```python
from build123d import *

# Parameters (mm, degrees)
F0_W     = 40
F0_H     = 30
F1_DEPTH = 7.5
F2_W     = 21.86022
F2_H     = 7.61192
F3_DEPTH = 25
F4_R     = 1.8
F5_DEPTH = 20


with BuildPart() as f1:
    # F0 (on Top) → F1 (new body, symmetric)
    with BuildSketch(Plane.XY):
        Rectangle(F0_W, F0_H)
    extrude(amount=F1_DEPTH, both=True)

    # F2 (on face) → F3 (cut)
    with BuildSketch(Plane.XY.offset(7.5)):
        with Locations((-9.06989, 0)):
            Rectangle(F2_W, F2_H)
    extrude(amount=-F3_DEPTH, mode=Mode.SUBTRACT)

    # F4 (on face) → F5 (cut)
    with BuildSketch(Plane.XY.offset(7.5)):
        with Locations((-15.035771, -10)):
            Circle(F4_R)
        with Locations((-15.035771, 10)):
            Circle(F4_R)
    extrude(amount=-F5_DEPTH, mode=Mode.SUBTRACT)


solid = f1.part
```
Geometry: final body of the model. Coordinates: model frame, mm. A direction names the side the tool comes from. Round coordinates to 2 decimals unless told otherwise and drop trailing zeros. Order: outer loops, then holes, each group sorted by start corner. A loop starts at its lowest first (then second) coordinate and runs counter-clockwise, first axis right, second up. Notation, with made-up numbers: (13.25, 32.25) -> (65.25, 32.25) arc R29 cw to (65.25, 68.25) -> close; hole circle Ø5 at (14.5, 83.5). An arc over 180 degrees is marked (long way). Write each question's results on one line, items separated by ' | '.
Q1. Section query A-A (y = -10). Output: boundary loops of the cut face in (x, z).
Response values:
outline: (-20, -7.5) -> (-16.84, -7.5) -> (-16.84, 7.5) -> (-20, 7.5) -> close; (-13.24, -7.5) -> (20, -7.5) -> (20, 7.5) -> (-13.24, 7.5) -> close
Q2. Pull-direction query (Y, two-part tool) for faces 3 (the face through (-16.834, 10.079, 0.105)), 4 (the face through (1.86, 0, 0)), 5 (the face through (0, 15, 0)), 6 (the face through (4, 0, 7.5)); classes: released by +Y, released by -Y, zero draft, split by the parting line, or undercut.
Response values:
face 3: undercut | face 4: undercut | face 5: released by +Y | face 6: zero draft
Q3. Section query B-B (z = -4.5). Output: boundary loops of the cut face in (x, y), and give its area (3 significant figures).
Response values:
outline: (-20, -15) -> (20, -15) -> (20, 15) -> (-20, 15) -> (-20, 3.81) -> (1.86, 3.81) -> (1.86, -3.81) -> (-20, -3.81) -> close; hole circle Ø3.6 at (-15.04, -10); hole circle Ø3.6 at (-15.04, 10) | area: 1,010 mm²
Q4. Section query D-D (y = 2). Output: boundary loops of the cut face in (x, z), and give its area (3 significant figures).
Response values:
outline: (1.86, -7.5) -> (20, -7.5) -> (20, 7.5) -> (1.86, 7.5) -> close | area: 272 mm²
Q5. Ray query, line 1 along Y through (x, z) = (-9, 2.25); line 2 along X through (y, z) = (-2, 2.5); line 3 along X through (y, z) = (9.5, 7.25). Return the intervals inside material, ascending.
Response values:
line 1: -15 to -3.81, 3.81 to 15 | line 2: 1.86 to 20 | line 3: -20 to -16.76, -13.31 to 20
Q6. Access query for faces 1 (the face through (-9, -3.806, 0)), 2 (the face through (-20, 9, 0)). Directions: +Z, -Z, +X, -X, +Y, -Y. A direction counts if a zero-diameter tool reaches every point of the face in a straight line with its end or side. Return the directions, or none.
Response values:
face 1: +Z, -Z, -X | face 2: +Z, -Z, -X, +Y, -Y
Q7. Section query C-C (x = -1.5). Output: boundary loops of the cut face in (y, z).
Response values:
outline: (-15, -7.5) -> (-3.81, -7.5) -> (-3.81, 7.5) -> (-15, 7.5) -> close; (3.81, -7.5) -> (15, -7.5) -> (15, 7.5) -> (3.81, 7.5) -> close
